from build123d import *

# Parameters (mm, degrees)
F0_R      = 16.002
F1_DEPTH  = 2.032
F3_R      = 12.827
F3_R_2    = 11.2268
F4_DEPTH  = 0.254
F2_R      = 1.5875
F5_DEPTH  = 2.032
F6_R      = 5.55625
F7_DEPTH  = 0.254
F8_R      = 3.175
F9_DEPTH  = 0.762
F10_R     = 0.381
F11_DEPTH = 0.508
F12_DEPTH = 14.2875


with BuildPart() as f1:
    # F0 (on Front) → F1 (new body)
    with BuildSketch(Plane.XZ):
        Circle(F0_R)
    extrude(amount=-F1_DEPTH)

    # F3 (on face) → F4 (cut)
    with BuildSketch(Plane.XZ):
        Circle(F3_R)
        Circle(F3_R_2, mode=Mode.SUBTRACT)
    extrude(amount=-F4_DEPTH, mode=Mode.SUBTRACT)

    # F2 (on face) → F5 (cut)
    with BuildSketch(Plane.XZ):
        with Locations((0, -7.9695228487)):
            Circle(F2_R)
        with Locations((-5.8604669757, -4.9584284425)):
            Circle(F2_R)
        with BuildLine():
            Line((-6.7264510825, 0), (-9.9014510825, 0))
            ThreePointArc((-9.9014510825, 0), (-8.3139510825, -1.5875), (-6.7264510825, 0))
        make_face()
        with BuildLine():
            ThreePointArc((-6.7264510825, 0), (-8.3139510825, 1.5875), (-9.9014510825, 0))
            Line((-9.9014510825, 0), (-6.7264510825, 0))
        make_face()
        with Locations((-5.4118158296, 5.3960969672)):
            Circle(F2_R)
        with Locations((0, 7.9223643988)):
            Circle(F2_R)
        with Locations((5.3672702052, 5.5701895617)):
            Circle(F2_R)
        with BuildLine():
            Line((6.2692415476, 0), (9.4442415476, 0))
            ThreePointArc((9.4442415476, 0), (7.8567415476, 1.5875), (6.2692415476, 0))
        make_face()
        with BuildLine():
            ThreePointArc((6.2692415476, 0), (7.8567415476, -1.5875), (9.4442415476, 0))
            Line((9.4442415476, 0), (6.2692415476, 0))
        make_face()
        with Locations((5.607039202, -5.3108036518)):
            Circle(F2_R)
    extrude(amount=-F5_DEPTH, mode=Mode.SUBTRACT)

    # F6 (on face) → F7 (join)
    with BuildSketch(Plane.XZ):
        Circle(F6_R)
    extrude(amount=F7_DEPTH)

    # F8 (on face) → F9 (join)
    with BuildSketch(Plane.XZ.offset(0.254)):
        Circle(F8_R)
    extrude(amount=F9_DEPTH)

    # F10 (on face) → F11 (join)
    with BuildSketch(Plane.XZ.offset(1.016)):
        with Locations((-1.543693963, 0)):
            Circle(F10_R)
        with Locations((-0.9479312136, 0.8902023229)):
            Circle(F10_R)
        with Locations((0, 1.2909881785)):
            Circle(F10_R)
        with Locations((0.9910054901, 0.9551946484)):
            Circle(F10_R)
        with Locations((1.4676158223, 0)):
            Circle(F10_R)
        with Locations((1.0343337624, -0.9079179104)):
            Circle(F10_R)
        with Locations((0, -1.3411998874)):
            Circle(F10_R)
        with Locations((-1.0887479328, -0.9079179104)):
            Circle(F10_R)
    extrude(amount=F11_DEPTH)

    # F12 (add): faces of the model
    f12_faces = [f1.faces().sort_by_distance(p)[0] for p in [
        (-15.5493950915, 0, 0),
        (-12.4641976527, 0.254, 0),
    ]]
    extrude(f12_faces, amount=F12_DEPTH)


solid = f1.part
Work out the finished part from the listing and answer in its coordinate system (mm). A direction names the side the tool comes from. Round coordinates to 2 decimals unless told otherwise and drop trailing zeros. Loops run counter-clockwise (first coordinate to the right, second up) from the corner with the lowest first, then second, coordinate; pieces in that order, holes last. Notation, with made-up numbers: (-10, -1.5) - (8, -1.5) arc R26 ccw to (8, 30.5) - close; hole circle Ø1 at (-18.75, 26). An arc over 180 degrees is marked (long way). Use one line per item in the form item = value. Start each with the question number.
(1) Determine the mould class of faces 3 (the face through (4.437, 1.002, -4.238)), 4 (the face through (0, 2.032, 0)) for opening direction X: +X half, -X half, draft (parallel to the pull), parting line (faces both ways), or undercut.
(2) Consider line 1 (Z direction, x = 0, y = 1.25); line 2 (X direction, y = 0.25, z = 5.5); line 3 (Y direction, x = -3, z = 7). Determine where each line is inside the solid, lowest interval first.
(3) Find section A-A on x = 10. Determine the outline of the cut face in (y, z).
(4) Which of the six approach directions +Z, -Z, +X, -X, +Y, -Y give full straight-line access (tool end or side, diameter ignored) to faces 1 (the face through (-0.69, -0.63, -3.1)), 2 (the face through (-6.8, 1, 0.48))?
(5) Find section B-B on y = -3.25. Determine the outline of the cut face in (x, z).
(6) Flat-ended cylindrical pins translate along their axes: P1, Ø12, axis at x = 3.5, z = 10.5, coming from the -Y side; P2, Ø3, axis at x = -8.31, z = 0, coming from the -Y side; P3, Ø1, axis at x = 7.5, y = -9, coming from the -Z side; P4, Ø13, axis at x = -2, z = 2, coming from the -Y side. Find the tip coordinate at first contact, or state that the pin passes through.
Answer list:
q1.face_3 = undercut
q1.face_4 = draft
q2.line_1 = -16 to -9.56, -6.38 to 6.33, 9.51 to 16
q2.line_2 = -15.03 to -7, -3.83 to 3.78, 6.95 to 15.03
q2.line_3 = 0 to 2.03
q3.outline = (-14.29, -12.49) - (2.03, -12.49) - (2.03, 12.49) - (-14.29, 12.49) - (-14.29, 8.03) - (-14.03, 8.03) - (-14.03, 5.1) - (0, 5.1) - (0, -5.1) - (-14.03, -5.1) - (-14.03, -8.03) - (-14.29, -8.03) - close
q4.face_1 = -Y
q4.face_2 = +Y, -Y
q5.outline = circle Ø32 at (0, 0); hole circle Ø22.45 at (0, 0)
q6.P1 = -14.29
q6.P2 = through
q6.P3 = -14.39
q6.P4 = -1.52
